Work out the finished part from the listing and answer in its coordinate system (mm). Face numbers are marked on the shaded views. A direction names the side the tool comes from. Round coordinates to 2 decimals unless told otherwise and drop trailing zeros. Write each loop counter-clockwise with the first axis right and the second up, starting at its lowest first coordinate (ties: lowest second). Pieces come first, ordered by that corner, then holes. Notation, with made-up numbers: (39, 83.25) -> (50, 83.25) arc R38 cw to (50, 121.25) -> close; hole circle Ø2 at (42, 80). An arc over 180 degrees is marked (long way). One line per item, written item: value.
```python
from build123d import *

# Parameters (mm, degrees)
BOSS_EXTRUDE1_DEPTH = 5


with BuildPart() as part:
    # Sketch1 → Boss-Extrude1 (new body)
    with BuildSketch(Plane(origin=(0, 0, 0), x_dir=(0, 0, -1), z_dir=(1, 0, 0))):
        with BuildLine():
            ThreePointArc((4.714045208, 16.666666667), (0, 20), (-4.714045208, 16.666666667))
            Line((-4.714045208, 16.666666667), (-9.428090416, 3.333333333))
            ThreePointArc((-9.428090416, 3.333333333), (0, -10), (9.428090416, 3.333333333))
            Line((9.428090416, 3.333333333), (4.714045208, 16.666666667))
        make_face()
        with BuildLine():
            ThreePointArc((2, 4.582575695), (0, -5), (-2, 4.582575695))
            Line((-2, 4.582575695), (-2, 6.802065863))
            Line((-2, 6.802065863), (2, 6.802065863))
            Line((2, 6.802065863), (2, 4.582575695))
        make_face(mode=Mode.SUBTRACT)
    extrude(amount=BOSS_EXTRUDE1_DEPTH)


solid = part.part
```
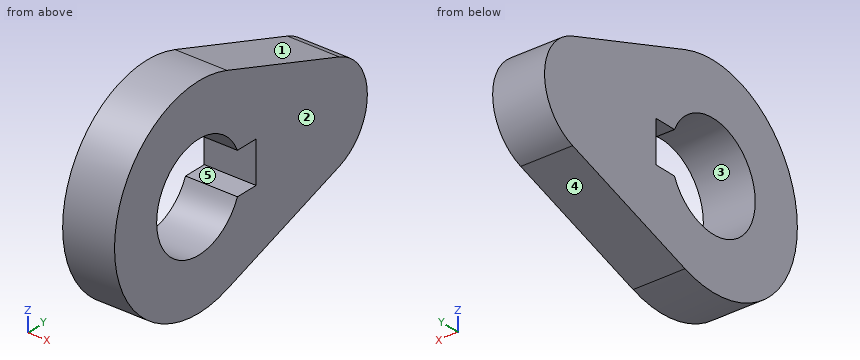
(1) A tool of negligible diameter and unlimited length cuts with its end or side. For the marked faces 4 and 5, from which of +Z, -Z, +X, -X, +Y, -Y can it reach the whole face along a straight path? Write none if from no direction.
Reported:
face 4: -Z, +X, -X, +Y
face 5: +X, -X
(2) Find section B-B on y = 0. Give the vertices of the cut face in (x, z), plus the area to 3 significant figures.
Reported:
outline: (0, -10) -> (5, -10) -> (5, -5) -> (0, -5) -> close; (0, 5) -> (5, 5) -> (5, 10) -> (0, 10) -> close
area: 50.0 mm2
(3) Flat-ended cylindrical pins translate along their axes: pin 1 Ø0.7 at (x, y) = (2, 5.5) entering from -Z; pin 2 Ø2.5 at (x, y) = (3.5, 5) entering from +Z; pin 3 Ø2 at (x, y) = (4.5, 8) entering from +Z. Find the tip coordinate at first contact, or state that the pin passes through.
Reported:
pin 1: stops at z = -8.79
pin 2: stops at z = 9.28
pin 3: stops at z = 8.13
(4) Find section D-D on z = -6. Give the vertices of the cut face in (x, y).
Reported:
outline: (0, -8) -> (5, -8) -> (5, 13.03) -> (0, 13.03) -> close
(5) Consider probe 1 along Y at (x, z) = (3.05, 0); probe 2 along Z at (x, y) = (1.5, 0); probe 3 along Y at (x, z) = (2.9, 1). Determine where each line is inside the solid, lowest interval first.
Reported:
probe 1: y = -10 to -5, 6.8 to 20
probe 2: z = -10 to -5, 5 to 10
probe 3: y = -9.95 to -4.9, 6.8 to 19.9
(6) Find section C-C on x = 0.65. Give the vertices of the cut face in (y, z), plus the area to 3 significant figures.
Reported:
outline: (3.33, -9.43) -> (16.67, -4.71) arc R5 ccw to (16.67, 4.71) -> (3.33, 9.43) arc R10 ccw (long way) to start; hole (4.58, -2) -> (6.8, -2) -> (6.8, 2) -> (4.58, 2) arc R5 ccw (long way) to start
area: 348 mm2
(7) Find section A-A on z = 0. Give the vertices of the cut face in (x, y), plus the area to 3 significant figures.
Reported:
outline: (0, -10) -> (5, -10) -> (5, -5) -> (0, -5) -> close; (0, 6.8) -> (5, 6.8) -> (5, 20) -> (0, 20) -> close
area: 91.0 mm2
(8) For a pull along Z with two mould halves and no side action, classify the marked faces 1, 2 and 3 as pulls with the +Z half, pulls with the -Z half, needs draft (parallel to the pull), parting line crosses it, or undercut.
Reported:
face 1: pulls with the +Z half
face 2: needs draft
face 3: undercut
